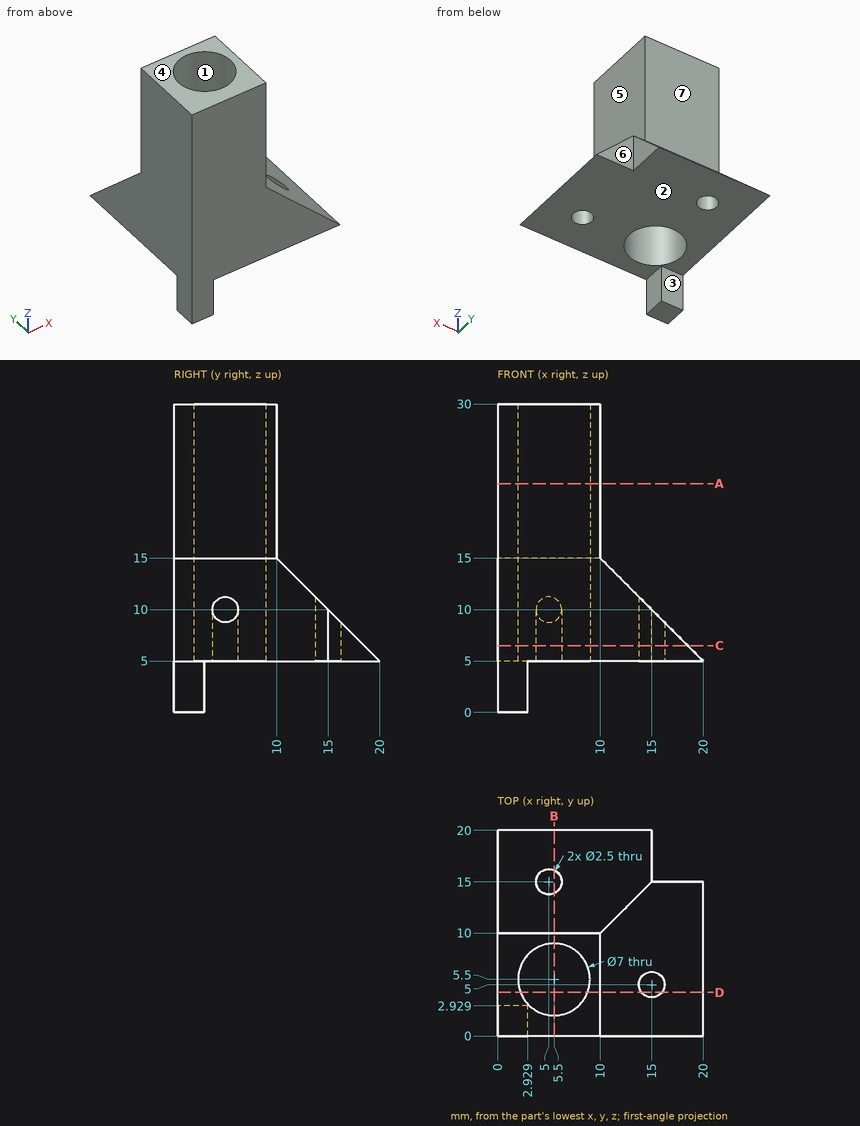
Can you work these out from the drawing? Everything is in mm from the part's minimum corner. A direction names the side the tool comes from. Give positions to 0.01 mm unless a question says otherwise; leave off trailing zeros. Order: outer loops, then holes, each group sorted by start corner. A loop starts at its lowest first (then second) coordinate and runs counter-clockwise, first axis right, second up.
Item 1: I need wall thicknesses on line 1 (X direction, y = 5, z = 6.75); line 2 (Y direction, x = 5, z = 8.5); line 3 (Y direction, x = 5, z = 7.75). Which ranges of each line are inside material? Lowest first, please.
Item 2: For the marked faces 4, 5, 6 and 7, which set-ups out of +Z, -Z, +X, -X, +Y, -Y let a thin tool reach every point of the face, with its end or its side?
Item 3: If we section it at A-A, the plane z = 22.25: Write out the boundary of the cut face in (x, y), plus the area to 3 significant figures.
Item 4: If we section it at D-D, the plane y = 4.25: Write out the boundary of the cut face in (x, z).
Item 5: I'm going to push flat-ended pins straight in: pin 1 (3 mm diameter, centred on x = 6, z = 19.5, fed in from +Y); pin 2 (1.5 mm diameter, centred on y = 16.5, z = 7.5, fed in from +X); pin 3 (0.9 mm diameter, centred on x = 1.5, z = 3, fed in from +Y). Where does each tip first touch, or does it pass through?
Item 6: If we section it at C-C, the plane z = 6.5: Write out the boundary of the cut face in (x, y).
Item 7: If we mould it in two halves opening along Y, with no side actions, what happens to the marked faces 1, 2 and 3? For each: pulls with the +Y half, pulls with the -Y half, needs draft (parallel to the pull), parting line crosses it, or undercut.
Item 8: If we section it at B-B, the plane x = 5.5: Write out the boundary of the cut face in (y, z).
Values:
1. line 1: x = 0 to 2.04, 8.96 to 13.75, 16.25 to 18.25
1. line 2: y = 0 to 2.04, 8.96 to 13.75, 16.25 to 16.5
1. line 3: y = 0 to 2.04, 8.96 to 13.75, 16.25 to 17.25
2. face 4: +Z, +X, -X, +Y, -Y
2. face 5: +Z, +X, +Y, -Y
2. face 6: +Z, -Z, +X, +Y
2. face 7: +Z, +X, -X, +Y
3. outline: (0, 0) - (10, 0) - (10, 10) - (0, 10) - close; hole circle Ø7 at (5.5, 5.5)
3. area: 61.5 mm2
4. outline: (0, 5) - (2.23, 5) - (2.23, 30) - (0, 30) - close; (8.77, 5) - (14, 5) - (14, 11) - (10, 15) - (10, 30) - (8.77, 30) - close; (16, 5) - (20, 5) - (16, 9) - close
5. pin 1: stops at y = 10
5. pin 2: stops at x = 15
5. pin 3: stops at y = 2.93
6. outline: (0, 0) - (18.5, 0) - (18.5, 15) - (15, 15) - (15, 18.5) - (0, 18.5) - close; hole circle Ø7 at (5.5, 5.5); hole circle Ø2.5 at (5, 15); hole circle Ø2.5 at (15, 5)
7. face 1: undercut
7. face 2: needs draft
7. face 3: pulls with the +Y half
8. outline: (0, 5) - (2, 5) - (2, 30) - (0, 30) - close; (9, 5) - (13.85, 5) - (13.85, 11.15) - (10, 15) - (10, 30) - (9, 30) - close; (16.15, 5) - (20, 5) - (16.15, 8.85) - close
